from build123d import *

# Parameters (mm, degrees)
SKETCH2_W               = 27.9908
SKETCH2_H               = 27.9908
CUT_EXTRUDE1_DEPTH      = 2.3876
CUT_EXTRUDE1_DEPTH_BACK = 2.3876


with BuildPart() as part:
    # Sketch1 → Revolve1 (revolve)
    with BuildSketch(Plane(origin=(0, 0, 0), x_dir=(0, 0, -1), z_dir=(1, 0, 0))):
        Polygon((-1.1938, 0), (-1.1938, 6.9977), (-0.684409098, 8.39724), (1.1938, 8.39724), (1.1938, 0), align=None)
    revolve(axis=Axis((0, 0, -1.1938), (0, 0, 1)))

    # Sketch2 → Cut-Extrude1 (cut, two sides)
    with BuildSketch(Plane.XY) as cut_extrude1_sk:
        Rectangle(SKETCH2_W, SKETCH2_H)
        Polygon((-8.001, 0), (-4.040123979, -6.9977), (4.040123979, -6.9977), (8.001, 0), (4.040123979, 6.9977), (-4.040123979, 6.9977), align=None, mode=Mode.SUBTRACT)
    extrude(amount=CUT_EXTRUDE1_DEPTH, mode=Mode.SUBTRACT)
    extrude(cut_extrude1_sk.sketch, amount=-CUT_EXTRUDE1_DEPTH_BACK, mode=Mode.SUBTRACT)

    # Sketch3 → Cut-Revolve1 (revolve, cut)
    with BuildSketch(Plane(origin=(0, 0, 0), x_dir=(0, 0, -1), z_dir=(1, 0, 0))):
        Polygon((-1.1938, 0), (-1.1938, 5.9944), (-0.2524, 5.053), (0.2524, 5.053), (1.1938, 5.9944), (1.1938, 0), align=None)
    revolve(axis=Axis((0, 0, -1.1938), (0, 0, 1)), mode=Mode.SUBTRACT)


solid = part.part
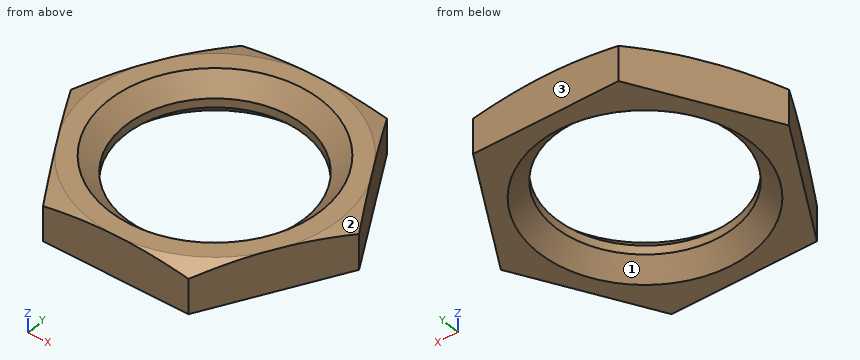
Verification items for the finished model (mm, model axes). Face numbers are marked on the shaded views. Give positions to 0.01 mm unless a question says otherwise; leave off trailing zeros. Write each loop counter-clockwise with the first axis right and the second up, starting at its lowest first coordinate (ties: lowest second). Pieces come first, ordered by that corner, then holes. Notation, with made-up numbers: M -19.5,37.5 L 14.5,37.5 A20 ccw 14.5,58.5 Z; hole C 86,27.5 d11. An arc over 180 degrees is marked long. Write item = value, one per line.
(1) Material ranges on line 1 (Y direction, x = 0, z = -0.1); line 2 (X direction, y = -2.5, z = 0.5); line 3 (X direction, y = -0.75, z = -0.55), recorded low to high.
Found:
line_1 = -7 to -5.05, 5.05 to 7
line_2 = -6.59 to -4.67, 4.67 to 6.59
line_3 = -7.58 to -5.3, 5.3 to 7.58
(2) Sectioned sample at A-A (z = -0.05). Record the cut outline in (x, y).
Found:
outline = M -8,0 L -4.04,-7 L 4.04,-7 L 8,0 L 4.04,7 L -4.04,7 Z; hole C 0,0 d10.11
(3) Sectioned sample at B-B (z = -0.8). Record the cut outline in (x, y), then the cut area to 3 significant figures.
Found:
outline = M -8,0 L -4.04,-7 L 4.04,-7 L 8,0 L 4.04,7 L -4.04,7 Z; hole C 0,0 d11.2
area = 70.0 mm2
(4) Draft check along Y on the marked faces 1, 2 and 3. Enter one of: released by +Y, released by -Y, zero draft, split by the parting line, or undercut.
Found:
face_1 = undercut
face_2 = split by the parting line
face_3 = released by +Y
